Here's how the part is built. I have some questions about the finished solid (model axes, mm). A direction names the side the tool comes from. Round coordinates to 2 decimals unless told otherwise and drop trailing zeros. Order: outer loops, then holes, each group sorted by start corner. A loop starts at its lowest first (then second) coordinate and runs counter-clockwise, first axis right, second up.
Autodesk Inventor part; units mm, degrees
ref_plane "YZ Plane" through (0, 0, 0) normal (1, 0, 0) x (0, 1, 0)
ref_plane "XZ Plane" through (0, 0, 0) normal (0, 1, 0) x (-1, 0, 0)
ref_plane "XY Plane" through (0, 0, 0) normal (0, 0, 1) x (1, 0, 0)
sketch "Sketch1" plane through (0, 0, 0) normal (0, 0, 1) x (1, 0, 0)
  line L0 (-33.7638, 59.8408) -> (17.0362, 59.8408)
  line L1 (17.0362, 59.8408) -> (17.0362, -16.3592)
  line L2 (17.0362, -16.3592) -> (-33.7638, -16.3592)
  line L3 (-33.7638, -16.3592) -> (-33.7638, 59.8408)
  dimension "d0" = 50.8
  dimension "d1" = 76.2
extrude "Extrusion1" add sketch "Sketch1" along normal blind 8.89
sketch "Sketch2" plane through (0, 0, 8.89) normal (0, 0, 1) x (1, 0, 0)
  line L0 (17.0362, 59.8408) -> (17.0362, -16.3592)
  line L1 (-33.7638, 59.8408) -> (17.0362, 59.8408)
  line L2 (17.0362, -16.3592) -> (-33.7638, -16.3592)
  line L3 (9.4162, 59.8408) -> (9.4162, -16.3592)
  dimension "d4" = 7.62
extrude "Extrusion2" add sketch "Sketch2" along normal blind 19.05
sketch "Sketch3" plane through (0, 0, 8.89) normal (0, 0, 1) x (1, 0, 0)
  point P0 (9.4162, -16.3592)
  point P1 (-33.7638, -16.3592)
  point P2 (-9.6338, -8.7392)
  point P3 (-25.6982, -1.1192)
  dimension "d7" = 19.05
  dimension "d8" = 7.62
  dimension "d9" = 17.78
  dimension "d10" = 15.24
hole "Hole1" at (-9.6338, -8.7392, 8.89) at (-25.6982, -1.1192, 8.89) direction (0, 0, -1) diameter 2.54 depth 12.7 tip angle 118
sketch "Sketch4" plane through (0, 0, 8.89) normal (0, 0, 1) x (1, 0, 0)
  line L0 (9.4162, -16.3592) -> (9.4162, 59.8408)
  line L1 (-33.7638, 59.8408) -> (9.4162, 59.8408)
  line L2 (-15.9838, 59.8408) -> (-15.9838, 9.0408)
  line L3 (-15.9838, 9.0408) -> (-3.2838, 9.0408)
  line L4 (-3.2838, 9.0408) -> (-3.2838, 59.8408)
  dimension "d18" = 12.7
  dimension "d19" = 12.7
  dimension "d22" = 50.8
extrude "Extrusion3" add sketch "Sketch4" along normal up to surface (19.05 mm away)
sketch "Sketch5" plane through (0, 0, 8.89) normal (0, 0, 1) x (1, 0, 0)
  line L0 (-3.2838, 59.8408) -> (9.4162, 59.8408)
  line L1 (-3.2838, 59.8408) -> (-3.2838, 9.0408)
  circle A0 centre (3.0662, 53.4908) radius 2.074
  dimension "d24" = 6.35
  dimension "d25" = 6.35
extrude "Extrusion4" cut sketch "Sketch5" against normal up to next
properties part number "base"
1. If we section it at A-A, the plane z = 18.5: Write out the boundary of the cut face in (x, y).
Evaluation:
outline: (-15.98, 9.04) - (-3.28, 9.04) - (-3.28, 59.84) - (-15.98, 59.84) - close; (9.42, -16.36) - (17.04, -16.36) - (17.04, 59.84) - (9.42, 59.84) - close
2. On a 3-axis mill with a long thin cutter (end or side, diameter ignored), from which of +Z, -Z, +X, -X, +Y, -Y can I reach the whole of each face in a straight line? I mean faces 4 (the flat face through (-10, 9.041, 18)), 5 (the cylindrical face through (4.02, 51.65, 4.51)), 6 (the flat face through (-3.284, 34, 18)). Say none if no direction works.
Evaluation:
face 4: +Z, -X, -Y
face 5: +Z, -Z
face 6: +Z, +Y, -Y
3. If we section it at C-C, the plane y = 20: Write out the boundary of the cut face in (x, z), and give its area (3 significant figures).
Evaluation:
outline: (-33.76, 0) - (17.04, 0) - (17.04, 27.94) - (9.42, 27.94) - (9.42, 8.89) - (-3.28, 8.89) - (-3.28, 27.94) - (-15.98, 27.94) - (-15.98, 8.89) - (-33.76, 8.89) - close
area: 839 mm2
4. I'm going to push flat-ended pins straight in: P1, Ø6.5, axis at x = -12, z = 14, coming from the -Y side; P2, Ø10, axis at x = -15.5, y = -4.5, coming from the +Z side; P3, Ø5.5, axis at y = 39, z = 14, coming from the -X side. Where does each tip first touch, or does it pass through?
Evaluation:
P1: stops at y = 9.04
P2: stops at z = 8.89
P3: stops at x = -15.98
5. If we mould it in two halves opening along Y, with no side actions, what happens to faces 1 (the flat face through (-9, 59.841, 11)), 2 (the flat face through (-15.984, 35, 18)), 3 (the cylindrical face through (-24.46, -0.84, 4.38))? For each: released by +Y, released by -Y, zero draft, split by the parting line, or undercut.
Evaluation:
face 1: released by +Y
face 2: zero draft
face 3: undercut
6. If we section it at B-B, the plane y = -9: Write out the boundary of the cut face in (x, z).
Evaluation:
outline: (-33.76, 0) - (-10.88, 0) - (-10.88, 8.89) - (-33.76, 8.89) - close; (-8.39, 0) - (17.04, 0) - (17.04, 27.94) - (9.42, 27.94) - (9.42, 8.89) - (-8.39, 8.89) - close
7. I need wall thicknesses on probe 1 along X at (y, z) = (38.5, 14.25); probe 2 along Z at (x, y) = (-24, 54); probe 3 along Y at (x, z) = (-13, 17). Which ranges of each line are inside material? Lowest first, please.
Evaluation:
probe 1: x = -15.98 to -3.28, 9.42 to 17.04
probe 2: z = 0 to 8.89
probe 3: y = 9.04 to 59.84
8. If we section it at D-D, the plane y = -1: Write out the boundary of the cut face in (x, z), and give its area (3 significant figures).
Evaluation:
outline: (-33.76, 0) - (-26.96, 0) - (-26.96, 8.89) - (-33.76, 8.89) - close; (-24.43, 0) - (17.04, 0) - (17.04, 27.94) - (9.42, 27.94) - (9.42, 8.89) - (-24.43, 8.89) - close
area: 574 mm2
